Part model, mm, in its own coordinate system. Coordinates: 2 decimals unless noted, no trailing zeros. Order: outer loops, then holes, each group sorted by start corner. A loop starts at its lowest first (then second) coordinate and runs counter-clockwise, first axis right, second up. Notation, with made-up numbers: (84, 11) - (105, 11) arc R21 cw to (105, 38) - close; hole circle Ø2 at (-8.75, 41.5). An arc over 180 degrees is marked (long way). Use a Markdown table: item, result. Add a question column.
1) Wall check: L1, parallel to Z at x = 13, y = 4.25; L2, parallel to X at y = 2.1, z = -80.5. Give the ranges that are in metal, low to high. Write a range as [from, to].
2) Drop flat-ended pins along their axis: P1, Ø3, axis at x = 11.5, z = -27, coming from the -Y side; P2, Ø2, axis at x = 64, z = -82, coming from the +Y side. Give the stop position or say it passes through.
3) Saw through at B-B on y = 2.45. Count the separate pieces of the cut face and the enclosed holes in it, then the cut area to 3 significant figures.
4) Saw through at A-A on x = 36. List the corners of the cut face in (y, z).
```python
from build123d import *

# Parameters (mm, degrees)
SKETCH1_W           = 100
SKETCH1_H           = 92
BOSS_EXTRUDE1_DEPTH = 6
SKETCH6_W           = 10
SKETCH6_H           = 6
CUT_EXTRUDE1_DEPTH  = 4
SKETCH61_W          = 10
SKETCH61_H          = 6
CUT_EXTRUDE11_DEPTH = 4
SKETCH62_W          = 10
SKETCH62_H          = 6
CUT_EXTRUDE12_DEPTH = 4
SKETCH63_W          = 10
SKETCH63_H          = 6
CUT_EXTRUDE13_DEPTH = 4
FILLET1_R           = 5


with BuildPart() as part:
    # Sketch1 → Boss-Extrude1 (new body)
    with BuildSketch(Plane(origin=(0, 0, 0), x_dir=(1, 0, 0), z_dir=(0, 1, 0))):
        with Locations((50, 46)):
            Rectangle(SKETCH1_W, SKETCH1_H)
    extrude(amount=BOSS_EXTRUDE1_DEPTH)

    # Sketch6 → Cut-Extrude1 (cut, symmetric)
    with BuildSketch(Plane(origin=(84.232221392, 3, -39), x_dir=(1, 0, 0), z_dir=(0, -1, 0))):
        with Locations((0.767778608, -44)):
            Rectangle(SKETCH6_W, SKETCH6_H)
    cut_extrude1 = extrude(amount=CUT_EXTRUDE1_DEPTH, both=True, mode=Mode.SUBTRACT)

    # Sketch61 → Cut-Extrude11 (cut, symmetric)
    with BuildSketch(Plane(origin=(60.898888059, 3, -39), x_dir=(1, 0, 0), z_dir=(0, -1, 0))):
        with Locations((0.767778608, -44)):
            Rectangle(SKETCH61_W, SKETCH61_H)
    cut_extrude11 = extrude(amount=CUT_EXTRUDE11_DEPTH, both=True, mode=Mode.SUBTRACT)

    # Sketch62 → Cut-Extrude12 (cut, symmetric)
    with BuildSketch(Plane(origin=(37.565554726, 3, -39), x_dir=(1, 0, 0), z_dir=(0, -1, 0))):
        with Locations((0.767778608, -44)):
            Rectangle(SKETCH62_W, SKETCH62_H)
    cut_extrude12 = extrude(amount=CUT_EXTRUDE12_DEPTH, both=True, mode=Mode.SUBTRACT)

    # Sketch63 → Cut-Extrude13 (cut, symmetric)
    with BuildSketch(Plane(origin=(14.232221392, 3, -39), x_dir=(1, 0, 0), z_dir=(0, -1, 0))):
        with Locations((0.767778608, -44)):
            Rectangle(SKETCH63_W, SKETCH63_H)
    cut_extrude13 = extrude(amount=CUT_EXTRUDE13_DEPTH, both=True, mode=Mode.SUBTRACT)

    # Mirror1: Cut-Extrude1, Cut-Extrude11, Cut-Extrude12, Cut-Extrude13 across plane
    add(cut_extrude1.mirror(Plane(origin=(0, 0, -46), x_dir=(1, 0, 0), z_dir=(0, 0, -1))), mode=Mode.SUBTRACT)
    add(cut_extrude11.mirror(Plane(origin=(0, 0, -46), x_dir=(1, 0, 0), z_dir=(0, 0, -1))), mode=Mode.SUBTRACT)
    add(cut_extrude12.mirror(Plane(origin=(0, 0, -46), x_dir=(1, 0, 0), z_dir=(0, 0, -1))), mode=Mode.SUBTRACT)
    add(cut_extrude13.mirror(Plane(origin=(0, 0, -46), x_dir=(1, 0, 0), z_dir=(0, 0, -1))), mode=Mode.SUBTRACT)

    # Fillet1
    fillet1_edges = [part.edges().sort_by_distance(p)[0] for p in [
        (0, 3, -92),
        (100, 3, -92),
        (100, 3, 0),
        (0, 3, 0),
    ]]
    fillet(fillet1_edges, radius=FILLET1_R)


solid = part.part
```
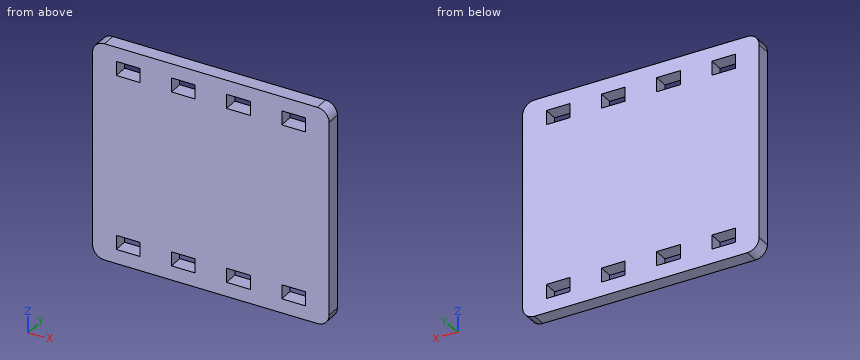
Results are:
| question | item | result |
|---|---|---|
| 1 | L1 | [-92, -86], [-80, -12], [-6, 0] |
| 1 | L2 | [0, 10], [20, 33.33], [43.33, 56.67], [66.67, 80], [90, 100] |
| 2 | P1 | y = 0 |
| 2 | P2 | through |
| 3 | separate pieces | 1 |
| 3 | enclosed holes | 8 |
| 3 | area | 8,700 mm2 |
| 4 | outline | (0, -92) - (6, -92) - (6, -86) - (0, -86) - close; (0, -80) - (6, -80) - (6, -12) - (0, -12) - close; (0, -6) - (6, -6) - (6, 0) - (0, 0) - close |
